Verification items for the finished model (mm, model axes). A direction names the side the tool comes from. Round coordinates to 2 decimals unless told otherwise and drop trailing zeros. Write each loop counter-clockwise with the first axis right and the second up, starting at its lowest first coordinate (ties: lowest second). Pieces come first, ordered by that corner, then holes. Notation, with made-up numbers: (-27, -32) - (-4, -32) arc R11 cw to (-4, -14) - close; hole circle Ø6 at (13.25, 9.25). An arc over 180 degrees is marked (long way). Answer as a JSON object with one key per item and string values.
```python
from build123d import *

# Parameters (mm, degrees)
EXTRUDE_1_DEPTH     = 12
EXTRUDE_3_DEPTH     = 6
SKETCH_4_R          = 2
EXTRUDE_4_DEPTH     = 4
CUT_EXTRUDE_2_DEPTH = 29.284271247
SKETCH_6_R          = 1.017604249
CUT_EXTRUDE_3_DEPTH = 38.312866414


with BuildPart() as part:
    # 草图1 → 凸台-拉伸1 (new body)
    with BuildSketch(Plane.XY):
        Polygon((-11, 12.536842105), (-16, 12.536842105), (-16, 14.536842105), (-11, 14.536842105), (-11, 16.036842105), (11, 16.036842105), (11, 14.536842105), (16, 14.536842105), (16, 12.536842105), (11, 12.536842105), (11, -5.463157895), (-11, -5.463157895), align=None)
    extrude(amount=EXTRUDE_1_DEPTH)

    # 草图2 → 凸台-拉伸3 (add)
    with BuildSketch(Plane(origin=(0, 16.036842105, 0), x_dir=(1, 0, 0), z_dir=(0, 1, 0))):
        with BuildLine():
            ThreePointArc((-0.479166667, -8.445144707), (11, -6), (-0.479166667, -3.554855293))
            ThreePointArc((-0.479166667, -3.554855293), (-3.5, -6), (-0.479166667, -8.445144707))
        make_face()
    extrude(amount=EXTRUDE_3_DEPTH)

    # 草图4 → 凸台-拉伸4 (add)
    with BuildSketch(Plane(origin=(0, 22.036842105, 0), x_dir=(1, 0, 0), z_dir=(0, 1, 0))):
        with Locations(Location((5, -6, 0), (0, 0, 180))):
            Circle(SKETCH_4_R)
    extrude(amount=EXTRUDE_4_DEPTH)

    # 草图5 → 切除-拉伸2 (cut, through all)
    with BuildSketch(Plane(origin=(0, 14.536842105, 0), x_dir=(-1, 0, 0), z_dir=(0, -1, 0))):
        with BuildLine():
            Line((-14.366025404, -6.458256145), (-16, -6.458256145))
            Line((-16, -6.458256145), (-16, -5.458256145))
            Line((-16, -5.458256145), (-14.366025404, -5.458256145))
            ThreePointArc((-14.366025404, -5.458256145), (-12.5, -5.958256145), (-14.366025404, -6.458256145))
        make_face()
        with BuildLine():
            Line((16, -6.458256145), (16, -5.458256145))
            Line((16, -5.458256145), (14.366025404, -5.458256145))
            ThreePointArc((14.366025404, -5.458256145), (12.5, -5.958256145), (14.366025404, -6.458256145))
            Line((14.366025404, -6.458256145), (16, -6.458256145))
        make_face()
    extrude(amount=CUT_EXTRUDE_2_DEPTH, mode=Mode.SUBTRACT)

    # 草图6 → 切除-拉伸3 (cut, through all)
    with BuildSketch(Plane(origin=(0, 26.036842105, 0), x_dir=(1, 0, 0), z_dir=(0, 1, 0))):
        with Locations(Location((5, -6, 0), (0, 0, 180))):
            Circle(SKETCH_6_R)
    extrude(amount=-CUT_EXTRUDE_3_DEPTH, mode=Mode.SUBTRACT)


solid = part.part
```
1. Go/stop test with flat-tipped pins: pin 1 (2.5 mm diameter, centred on x = 13, z = 3.5, fed in from +Y); pin 2 (3 mm diameter, centred on x = 7.5, z = 9.5, fed in from +Y); pin 3 (0.8 mm diameter, centred on y = 15.5, z = 4.5, fed in from +X). Record where each tip stops, or that it passes through.
Completed:
{"pin 1": "stops at y = 14.54", "pin 2": "stops at y = 22.04", "pin 3": "stops at x = 11"}
2. Material ranges on probe 1 along Z at (x, y) = (-13.5, 14.15); probe 2 along X at (y, z) = (4, 8.5); probe 3 along Y at (x, z) = (-3.5, 9.5), recorded low to high. Write a range as from..to.
Completed:
{"probe 1": "z = 0..4.96, 6.96..12", "probe 2": "x = -11..11", "probe 3": "y = -5.46..16.04"}
3. Access from +Z, -Z, +X, -X, +Y, -Y to the whole of each face (thin tool, end or side, straight path). Record for faces 1 (the face through (12, 14.537, 6)), 2 (the face through (-12, 12.537, 6)), 3 (the face through (-15, 14, 6.458)).
Completed:
{"face 1": "+Z, -Z, +X, +Y", "face 2": "+Z, -Z, -X, -Y", "face 3": "-X, +Y, -Y"}
4. Mould release check, pull along Z, two halves, no side actions. Record for faces 4 (the face through (6.474, 24.009, 7.352)), 5 (the face through (15, 14, 5.458)), 6 (the face through (16, 14, 3)): released by +Z, released by -Z, zero draft, split by the parting line, or undercut.
Completed:
{"face 4": "split by the parting line", "face 5": "undercut", "face 6": "zero draft"}
5. Cross-section at D-D (z = 10). Record the boundary of the cut face in (x, y), plus the area to 3 significant figures.
Completed:
{"outline": "(-16, 12.54) - (-11, 12.54) - (-11, -5.46) - (11, -5.46) - (11, 12.54) - (16, 12.54) - (16, 14.54) - (11, 14.54) - (11, 16.04) - (9.47, 16.04) - (9.47, 22.04) - (0.53, 22.04) - (0.53, 16.04) - (-11, 16.04) - (-11, 14.54) - (-16, 14.54) - close", "area": "547 mm^2"}
6. Cross-section at A-A (x = -13.5). Record the boundary of the cut face in (y, z).
Completed:
{"outline": "(12.54, 0) - (14.54, 0) - (14.54, 4.96) - (12.54, 4.96) - close; (12.54, 6.96) - (14.54, 6.96) - (14.54, 12) - (12.54, 12) - close"}
7. Cross-section at B-B (x = -1). Record the boundary of the cut face in (y, z).
Completed:
{"outline": "(-5.46, 0) - (16.04, 0) - (16.04, 3.5) - (22.04, 3.5) - (22.04, 8.5) - (16.04, 8.5) - (16.04, 12) - (-5.46, 12) - close"}
8. Cross-section at C-C (y = 6). Record the boundary of the cut face in (x, z).
Completed:
{"outline": "(-11, 0) - (11, 0) - (11, 12) - (-11, 12) - close; hole circle Ø2.04 at (5, 6)"}
